Part model, mm, in its own coordinate system. Give positions to 0.01 mm unless a question says otherwise; leave off trailing zeros. Loops run counter-clockwise (first coordinate to the right, second up) from the corner with the lowest first, then second, coordinate; pieces in that order, holes last. Notation, with made-up numbers: (-22, 70.5) -> (9, 70.5) arc R20 ccw to (9, 90.5) -> close; hole circle Ø10 at (11, 18.25). An arc over 180 degrees is marked (long way). Write item = value, one per line.
from build123d import *

# Parameters (mm, degrees)
F0_W      = 152.4
F0_H      = 63.5
F1_DEPTH  = 15.24
F2_SIZE   = 14.986
F1_FACE_W = 152.4
F1_FACE_H = 63.5
F3_DEPTH  = 14.986
F4_SIZE   = 14.986


with BuildPart() as f1:
    # F0 (on Top) → F1 (new body)
    with BuildSketch(Plane.XY):
        with Locations((-13.443335, 12.47429)):
            Rectangle(F0_W, F0_H)
    extrude(amount=F1_DEPTH)

    # F2
    f2_edges = [f1.edges().sort_by_distance(p)[0] for p in [
        (-13.443335, 44.22429, 15.24),
    ]]
    chamfer(f2_edges, length=F2_SIZE)

    # F1_face (on face) → F3 (join)
    with BuildSketch(Plane(origin=(-13.443335, 12.47429, 0), x_dir=(1, 0, 0), z_dir=(0, 0, -1))):
        Rectangle(F1_FACE_W, F1_FACE_H)
    extrude(amount=F3_DEPTH)

    # F4
    f4_edges = [f1.edges().sort_by_distance(p)[0] for p in [
        (-13.443335, 44.22429, -14.986),
    ]]
    chamfer(f4_edges, length=F4_SIZE)


solid = f1.part
1) Slice it at A-A, the plane x = 46.5. List the corners of the cut face in (y, z), and give its area (3 significant figures).
Resolved:
outline = (-19.28, -14.99) -> (29.24, -14.99) -> (44.22, 0) -> (44.22, 0.25) -> (29.24, 15.24) -> (-19.28, 15.24) -> close
area = 1,690 mm²
2) Slice it at B-B, the plane z = -8.5. List the corners of the cut face in (x, y), and give its area (3 significant figures).
Resolved:
outline = (-89.64, -19.28) -> (62.76, -19.28) -> (62.76, 35.72) -> (-89.64, 35.72) -> close
area = 8,380 mm²
3) Drop flat-ended pins along their axis: P1, Ø3, axis at x = -7.5, z = -2, coming from the +Y side; P2, Ø5, axis at x = -44.5, z = -9, coming from the +Y side. Give the stop position or say it passes through.
Resolved:
P1 = 43.72
P2 = 37.72
4) Pull direction X, two halves, no side cores. Call faces 1 (the face through (62.757, 6, 0)), 2 (the face through (-15, 5, -14.986)), 3 (the face through (-89.643, 6, 0)): pulls with the +X half, pulls with the -X half, needs draft (parallel to the pull), parting line crosses it, or undercut.
Resolved:
face_1 = pulls with the +X half
face_2 = needs draft
face_3 = pulls with the -X half
5) Drill centre lines: line 1 along Y through (x, z) = (1.5, 9.5); line 2 along Y through (x, z) = (-28.5, -9.5). Where is each one in solid material? Low to high. Write a range as [from, to].
Resolved:
line_1 = [-19.28, 34.98]
line_2 = [-19.28, 34.72]
6) Slice it at C-C, the plane y = 34. List the corners of the cut face in (x, z), and give its area (3 significant figures).
Resolved:
outline = (-89.64, -10.22) -> (62.76, -10.22) -> (62.76, 10.48) -> (-89.64, 10.48) -> close
area = 3,160 mm²
